from build123d import *

# Parameters (mm, degrees)
F0_W        = 152.4
F0_H        = 203.2
F1_DEPTH    = 9.525
F2_W        = 88.9
F2_H        = 88.9
F3_DEPTH    = 762
F4_R        = 7.14375
F5_DEPTH    = 25.4
F7_T        = 4.7625
F7_T3_DEPTH = 98.425
F7_T5_DEPTH = 98.425
F6_R        = 6.35
F8_DEPTH    = 25.4


# Not quite as in the source:
# - a shell that OpenCascade refuses in one call is made with other operations: the cavity is built on its own and cut out


with BuildPart() as f1:
    # F0 (on Top) → F1 (new body)
    with BuildSketch(Plane.XY):
        with Locations((76.2, 101.6)):
            Rectangle(F0_W, F0_H)
    extrude(amount=F1_DEPTH)

    # F2 (on face) → F3 (join)
    with BuildSketch(Plane.XY.offset(9.525)):
        with Locations((76.2, 101.6)):
            Rectangle(F2_W, F2_H)
    extrude(amount=F3_DEPTH)

    # F4 (on face) → F5 (cut)
    with BuildSketch(Plane.XY.offset(9.525)):
        with Locations((127, 177.8)):
            Circle(F4_R)
        with Locations((127, 25.4)):
            Circle(F4_R)
        with Locations((25.4, 25.4)):
            Circle(F4_R)
        with Locations((25.4, 177.8)):
            Circle(F4_R)
    extrude(amount=-F5_DEPTH, mode=Mode.SUBTRACT)

    # F7: shell of thickness 4.7625, made by hand


with BuildPart() as f7_core1:
    # F7_t2: copy of F1
    add(f1.part)

    # the walls: a layer under each face that stays
    f7_faces = [f7_core1.faces().sort_by_distance(p)[0] for p in [
        (0, 101.6, 4.7625),
        (76.2, 203.2, 4.7625),
        (76.2, 0, 4.7625),
        (76.2, 101.6, 0),
        (25.4, 33.8666666667, 9.525),
        (152.4, 101.6, 4.7625),
        (18.25625, 25.4, 4.7625),
        (119.85625, 25.4, 4.7625),
        (18.25625, 177.8, 4.7625),
        (119.85625, 177.8, 4.7625),
        (120.65, 101.6, 390.525),
        (76.2, 57.15, 390.525),
        (76.2, 146.05, 390.525),
        (31.75, 101.6, 390.525),
    ]]
    thicken(f7_faces, amount=-F7_T, mode=Mode.SUBTRACT)

    # F7_s4 → F7_t3 (cut)
    with BuildSketch(Plane.XZ.offset(-150.8125)):
        Polygon((120.697625, 9.572625), (120.65, 4.7625), (115.8875, 4.7625), (115.8875, 9.525), align=None)
        Polygon((31.702375, 9.572625), (31.75, 4.7625), (36.5125, 4.7625), (36.5125, 9.525), align=None)
    extrude(amount=F7_T3_DEPTH, mode=Mode.SUBTRACT)

    # F7_s6 → F7_t5 (cut)
    with BuildSketch(Plane.YZ.offset(26.9875)):
        Polygon((57.102375, 9.572625), (57.15, 4.7625), (61.9125, 4.7625), (61.9125, 9.525), align=None)
        Polygon((146.097625, 9.572625), (146.05, 4.7625), (141.2875, 4.7625), (141.2875, 9.525), align=None)
    extrude(amount=F7_T5_DEPTH, mode=Mode.SUBTRACT)


with BuildPart() as f1_1:
    add(f1.part)

    # what is left inside the walls is the cavity
    f7_cavity = [f7_core1.part.solids().sort_by_distance(p)[0] for p in [
        (36.560125, 88.370833, 388.14375),
    ]]
    add(f7_cavity, mode=Mode.SUBTRACT)

    # F6 (on face) → F8 (cut)
    with BuildSketch(Plane.XZ.offset(-57.15)):
        with Locations((76.2, 669.925)):
            Circle(F6_R)
        with Locations((76.2, 568.325)):
            Circle(F6_R)
    extrude(amount=-F8_DEPTH, mode=Mode.SUBTRACT)


solid = f1_1.part
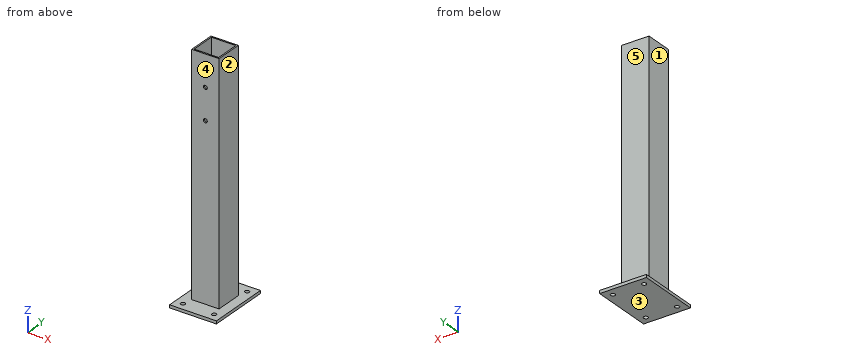
Could you check a few things on this model? Use its own coordinates, in mm. Face numbers are marked on the shaded views. A direction names the side the tool comes from. Round coordinates to 2 decimals unless told otherwise and drop trailing zeros. Order: outer loops, then holes, each group sorted by start corner. A loop starts at its lowest first (then second) coordinate and runs counter-clockwise, first axis right, second up.
(1) Please list where these lines run through material, in increasing order: line 1 along Y through (x, z) = (25.4, 6.25); line 2 along Z through (x, y) = (76.2, 59.3) (3 decimals); line 3 along Y through (x, z) = (77, 412.5).
Response values:
line 1: y = 0 to 18.26, 32.54 to 170.66, 184.94 to 203.2
line 2: z = 0 to 561.975, 574.675 to 663.575, 676.275 to 771.525
line 3: y = 57.15 to 61.91, 141.29 to 146.05
(2) I'm going to push flat-ended pins straight in: pin 1 (1 mm diameter, centred on y = 145.5, z = 689, fed in from -X); pin 2 (1 mm diameter, centred on x = 137, y = 91, fed in from +Z) (3 decimals); pin 3 (10 mm diameter, centred on x = 76.2, z = 669.925, fed in from -Y); pin 4 (11.5 mm diameter, centred on x = 25.4, y = 177.8, fed in from +Z). Where does each tip first touch, or does it pass through?
Response values:
pin 1: stops at x = 31.75
pin 2: stops at z = 9.525
pin 3: stops at y = 141.29
pin 4: passes through
(3) Imagine slicing it at A-A (z = 645). Write out the boundary of the cut face in (x, y).
Response values:
outline: (31.75, 57.15) - (120.65, 57.15) - (120.65, 146.05) - (31.75, 146.05) - close; hole (36.51, 61.91) - (115.89, 61.91) - (115.89, 141.29) - (36.51, 141.29) - close
(4) Imagine slicing it at B-B (y = 177.8). Write out the boundary of the cut face in (x, z) (3 decimals), plus the area to 3 significant figures.
Response values:
outline: (0, 0) - (18.256, 0) - (18.256, 9.525) - (0, 9.525) - close; (32.544, 0) - (119.856, 0) - (119.856, 9.525) - (32.544, 9.525) - close; (134.144, 0) - (152.4, 0) - (152.4, 9.525) - (134.144, 9.525) - close
area: 1,180 mm2
(5) Which directions (+Z, -Z, +X, -X, +Y, -Y) give clear straight access to the entire face, cutting with the end or side of a thin tool? Please do the marked faces 1, 2, 3, 4 and 5.
Response values:
face 1: +Z, -X, +Y, -Y
face 2: +Z, +X, +Y, -Y
face 3: -Z, +X, -X, +Y, -Y
face 4: +Z, +X, -X, -Y
face 5: +Z, +X, -X, +Y
